CAD build for the part. Positions are in the model's coordinates, mm. Face numbers are marked on the shaded views. A direction names the side the tool comes from. Give positions to 0.01 mm unless a question says otherwise; leave off trailing zeros. Loops run counter-clockwise (first coordinate to the right, second up) from the corner with the lowest first, then second, coordinate; pieces in that order, holes last. Notation, with made-up numbers: (42, -15) - (65, -15) arc R26 cw to (65, 24) - close; hole circle Ø9 at (-26, 35.25). An arc over 180 degrees is marked (long way). Return JSON: item names as keys, results as strings.
from build123d import *

# Parameters (mm, degrees)
SKETCH024_R           = 22
PAD011_DEPTH          = 80.15
PAD012_DEPTH          = 80.15
POLARPATTERN007_COUNT = 6
POCKET014_DEPTH       = 80.151


with BuildPart() as part:
    # Sketch024 → Pad011 (new body)
    with BuildSketch(Plane.XY):
        Circle(SKETCH024_R)
    extrude(amount=PAD011_DEPTH)

    # Sketch022 → Pad012 (join)
    with BuildSketch(Plane.XY):
        with BuildLine():
            ThreePointArc((39.721688, -1.5), (39.75, 0), (39.721688, 1.5))
            Line((21.424285, 5), (39.721688, 1.5))
            Line((21.424285, 5), (14.666667, 0))
            Line((14.666667, 0), (21.424285, -5))
            Line((21.424285, -5), (39.721688, -1.5))
        make_face()
    pad012 = extrude(amount=PAD012_DEPTH)

    # PolarPattern007: Pad012 ×6 about axis
    polarpattern007_axis = Axis((0, 0, 0), (0, 0, 1))
    for i in range(1, POLARPATTERN007_COUNT):
        add(pad012.rotate(polarpattern007_axis, i * 360 / POLARPATTERN007_COUNT))

    # Sketch023 → Pocket014 (cut, through all)
    with BuildSketch(Plane.XY):
        Polygon((14.3875, 8.306627), (0, 16.613254), (-14.3875, 8.306627), (-14.3875, -8.306627), (0, -16.613254), (14.3875, -8.306627), align=None)
    extrude(amount=POCKET014_DEPTH, mode=Mode.SUBTRACT)


with BuildPart() as part_1:
    # Body030 placement: moved
    add(part.part.moved(Location((0, -100, 0))))


solid = part_1.part
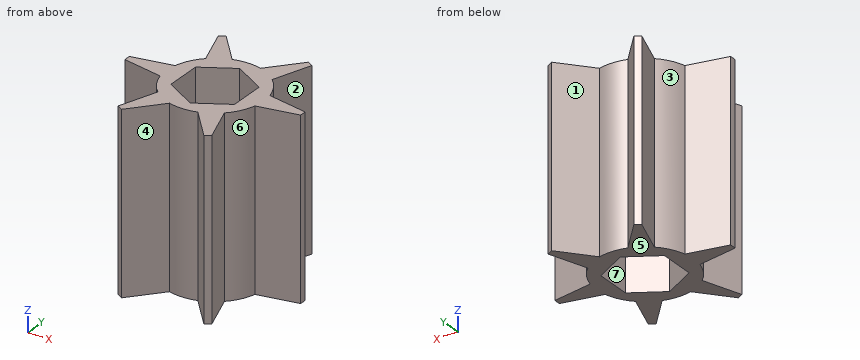
1. Drill centre lines: probe 1 along X at (y, z) = (-106, 36.5); probe 2 along X at (y, z) = (-77, 32); probe 3 along Y at (x, z) = (14, 31). Where is each one in solid material? Low to high.
Values follow:
{"probe 1": "x = -21.17 to -14.39, 14.39 to 21.17", "probe 2": "x = -17.46 to -8.06, 8.06 to 17.46", "probe 3": "y = -129.87 to -108.53, -91.47 to -70.13"}
2. Drop flat-ended pins along their axis: P1, Ø4, axis at x = -11.5, z = 47.5, coming from the +Y side; P2, Ø4, axis at x = -31.5, z = 45, coming from the +Y side; P3, Ø10, axis at x = 23, z = 47.5, coming from the -Y side. Give the stop position or say it passes through.
Values follow:
{"P1": "stops at y = -70.71", "P2": "stops at y = -96.54", "P3": "stops at y = -135.15"}
3. Cut at D-D, the plane x = -4. Write the cut outline in (y, z).
Values follow:
{"outline": "(-121.63, 0) - (-114.3, 0) - (-114.3, 80.15) - (-121.63, 80.15) - close; (-85.7, 0) - (-78.37, 0) - (-78.37, 80.15) - (-85.7, 80.15) - close"}
4. Cut at B-B, the plane y = -97. Write the cut outline in (x, z), plus the area to 3 significant figures.
Values follow:
{"outline": "(-31.88, 0) - (-14.39, 0) - (-14.39, 80.15) - (-31.88, 80.15) - close; (14.39, 0) - (31.88, 0) - (31.88, 80.15) - (14.39, 80.15) - close", "area": "2,800 mm²"}
5. Cut at C-C, the plane x = 20. Write the cut outline in (y, z), plus the area to 3 significant figures.
Values follow:
{"outline": "(-134.35, 0) - (-130.31, 0) - (-130.31, 80.15) - (-134.35, 80.15) - close; (-109.17, 0) - (-90.83, 0) - (-90.83, 80.15) - (-109.17, 80.15) - close; (-69.69, 0) - (-65.65, 0) - (-65.65, 80.15) - (-69.69, 80.15) - close", "area": "2,120 mm²"}
6. Which spindle directions (+Z, -Z, +X, -X, +Y, -Y) get a long thin tool onto all of the face, cutting with end or side? Do the marked faces 1, 2, 3 and 4. Say none if no direction does.
Values follow:
{"face 1": "+Z, -Z, +Y", "face 2": "+Z, -Z, +X", "face 3": "+Z, -Z, -X", "face 4": "+Z, -Z, -Y"}
7. Pull direction X, two halves, no side cores. Call the marked faces 5, 6 and 7: +X half, -X half, draft (parallel to the pull), parting line (faces both ways), or undercut.
Values follow:
{"face 5": "draft", "face 6": "+X half", "face 7": "undercut"}
